The listing builds one solid part. Answer for the finished solid, in the listing's coordinates (mm). A direction names the side the tool comes from. Coordinates: 2 decimals unless noted, no trailing zeros. Loops run counter-clockwise (first coordinate to the right, second up) from the corner with the lowest first, then second, coordinate; pieces in that order, holes last. Notation, with made-up numbers: (30, 40) - (87, 40) arc R19 cw to (87, 62) - close; hole circle Ø7 at (-22, 0.5). An arc over 180 degrees is marked (long way). Use one line per item in the form item = value. Start each with the question number.
Autodesk Inventor part; units mm, degrees
ref_plane "YZ Plane" through (0, 0, 0) normal (1, 0, 0) x (0, 1, 0)
ref_plane "XZ Plane" through (0, 0, 0) normal (0, 1, 0) x (-1, 0, 0)
ref_plane "XY Plane" through (0, 0, 0) normal (0, 0, 1) x (1, 0, 0)
sketch "Sketch1" plane through (0, 0, 0) normal (0, 0, 1) x (1, 0, 0)
  circle A0 centre (0, 0) radius 11
  circle A1 centre (0, 0) radius 2.5
  dimension "d0" = 22
  dimension "d1" = 5
extrude "Extrusion1" add sketch "Sketch1" along normal mid plane 2.8
sketch "Sketch2" plane through (0, 0, 1.4) normal (0, 0, 1) x (1, 0, 0)
  circle A0 centre (0, 0) radius 7.5 construction
  point P0 (-5.3033, 5.3033)
  point P1 (5.3033, 5.3033)
  point P2 (-5.3033, -5.3033)
  point P3 (5.3033, -5.3033)
  dimension "d4" = 15
  dimension "d5" = 90
hole "Hole1" at (-5.3033, 5.3033, 1.4) at (5.3033, 5.3033, 1.4) at (-5.3033, -5.3033, 1.4) at (5.3033, -5.3033, 1.4) direction (0, 0, -1) diameter 3 end through all
sketch "Sketch3" plane through (0, 0, 1.4) normal (0, 0, 1) x (1, 0, 0)
  circle A0 centre (0, 0) radius 4
  circle A1 centre (0, 0) radius 2.5
  dimension "d13" = 8
extrude "Extrusion2" add sketch "Sketch3" along normal blind 1
properties part number "shaftmount"
(1) A cutting plane is placed at A-A (y = 0). Determine the outline of the cut face in (x, z).
(2) For faces 5 (the face through (0, -5, 1.4)), 6 (the face through (5.88, -6.69, -0.02)), determine the directions among +Z, -Z, +X, -X, +Y, -Y from which every point of the face is accessible in a straight line to the end or side of a thin tool.
(3) A cutting plane is placed at C-C (x = -4.75). Determine the outline of the cut face in (y, z).
(4) Determine the mould class of faces 1 (the face through (0, 3, -1.4)), 2 (the face through (-0.54, -2.44, 0.53)), 3 (the face through (-0.867, 3.905, 1.893)), 4 (the face through (-6.57, 4.5, -0.02)) for opening direction Y: +Y half, -Y half, draft (parallel to the pull), parting line (faces both ways), or undercut.
(5) Each of these flat-tipped pins is pushed along its axis until it touches: pin 1 Ø4 at (x, y) = (-5.3, -5.3) entering from +Z; pin 2 Ø1.8 at (x, y) = (-5.3, 5.3) entering from -Z (3 decimals); pin 3 Ø1 at (x, z) = (-5, -0.5) entering from -Y. Where does it stop, or does it pass through?
(6) Find the intervals of material crossed by probe 1 along X at (y, z) = (-6.25, 0.85); probe 2 along Y at (x, z) = (0, -0.45); probe 3 along Z at (x, y) = (-5.75, -9.25), in increasing order. Write a range as from..to.
(7) A cutting plane is placed at D-D (z = -0.95). Determine the outline of the cut face in (x, y), then the cut area to 3 significant figures.
Evaluation:
q1.outline = (-11, -1.4) - (-2.5, -1.4) - (-2.5, 2.4) - (-4, 2.4) - (-4, 1.4) - (-11, 1.4) - close; (2.5, -1.4) - (11, -1.4) - (11, 1.4) - (4, 1.4) - (4, 2.4) - (2.5, 2.4) - close
q2.face_5 = +Z
q2.face_6 = +Z, -Z
q3.outline = (-9.92, -1.4) - (-6.7, -1.4) - (-6.7, 1.4) - (-9.92, 1.4) - close; (-3.91, -1.4) - (3.91, -1.4) - (3.91, 1.4) - (-3.91, 1.4) - close; (6.7, -1.4) - (9.92, -1.4) - (9.92, 1.4) - (6.7, 1.4) - close
q4.face_1 = draft
q4.face_2 = undercut
q4.face_3 = parting line
q4.face_4 = undercut
q5.pin_1 = 1.4
q5.pin_2 = through
q5.pin_3 = -10.04
q6.probe_1 = -9.05..-6.47, -4.14..4.14, 6.47..9.05
q6.probe_2 = -11..-2.5, 2.5..11
q6.probe_3 = -1.4..1.4
q7.outline = circle Ø22 at (0, 0); hole circle Ø3 at (-5.3, -5.3); hole circle Ø3 at (-5.3, 5.3); hole circle Ø5 at (0, 0); hole circle Ø3 at (5.3, -5.3); hole circle Ø3 at (5.3, 5.3)
q7.area = 332 mm^2
